The listing builds one solid part. Answer for the finished solid, in the listing's coordinates (mm). Face numbers are marked on the shaded views. A direction names the side the tool comes from. Give positions to 0.01 mm unless a question says otherwise; leave off trailing zeros. Loops run counter-clockwise (first coordinate to the right, second up) from the corner with the lowest first, then second, coordinate; pieces in that order, holes last. Notation, with made-up numbers: (86, -6.5) - (115, -6.5) arc R17 cw to (115, 2.5) - close; hole circle Ø2 at (39, -30.5). An arc over 180 degrees is marked (long way). One line per item, written item: value. Start each with the question number.
from build123d import *

# Parameters (mm, degrees)
SKETCH1_R           = 1.651
BOSS_EXTRUDE2_DEPTH = 6.35
SKETCH2_R           = 1.143
CUT_EXTRUDE1_DEPTH  = 7.35
SKETCH3_R           = 12.1285
CUT_EXTRUDE2_DEPTH  = 7.35
SKETCH4_W           = 28.562713242
SKETCH4_H           = 11.677503754
BOSS_EXTRUDE3_DEPTH = 6.35
SKETCH5_W           = 216.7214489
SKETCH5_H           = 130.569220634
CUT_EXTRUDE4_DEPTH  = 7.35
SKETCH11_R          = 3.937
CUT_EXTRUDE11_DEPTH = 7.35
SKETCH12_W          = 8.89
SKETCH12_H          = 8.89
CUT_EXTRUDE12_DEPTH = 7.35
SKETCH14_R          = 3.175
CUT_EXTRUDE14_DEPTH = 45.45
CUT_EXTRUDE15_DEPTH = 21.59
SKETCH16_R          = 12.192
CUT_EXTRUDE16_DEPTH = 21.59
SKETCH57_R          = 1.651
CUT_EXTRUDE57_DEPTH = 58.674


with BuildPart() as part:
    # Sketch1 → Boss-Extrude2 (new body)
    with BuildSketch(Plane.XY):
        with BuildLine():
            Line((-64.964441474, 37.338), (-54.550441474, 37.338))
            Line((-54.550441474, 37.338), (-54.550441474, -37.338))
            Line((-54.550441474, -37.338), (-64.964441474, -37.338))
            ThreePointArc((-64.964441474, -37.338), (0, -74.93), (64.964441474, -37.338))
            Line((64.964441474, -37.338), (54.550441474, -37.338))
            Line((54.550441474, -37.338), (54.550441474, 37.338))
            Line((54.550441474, 37.338), (64.964441474, 37.338))
            ThreePointArc((64.964441474, 37.338), (0, 74.93), (-64.964441474, 37.338))
        make_face()
        with Locations((-46.482, 11.049)):
            Circle(SKETCH1_R, mode=Mode.SUBTRACT)
        with Locations((-21.083270032, 10.795)):
            Circle(SKETCH1_R, mode=Mode.SUBTRACT)
        with Locations((-21.083270032, -10.795)):
            Circle(SKETCH1_R, mode=Mode.SUBTRACT)
        with Locations((-46.482, -11.049)):
            Circle(SKETCH1_R, mode=Mode.SUBTRACT)
        with Locations((46.482, -11.049)):
            Circle(SKETCH1_R, mode=Mode.SUBTRACT)
        with Locations((21.083270032, -10.795)):
            Circle(SKETCH1_R, mode=Mode.SUBTRACT)
        with Locations((21.083270032, 10.795)):
            Circle(SKETCH1_R, mode=Mode.SUBTRACT)
        with Locations((46.482, 11.049)):
            Circle(SKETCH1_R, mode=Mode.SUBTRACT)
    extrude(amount=BOSS_EXTRUDE2_DEPTH)

    # Sketch2 → Cut-Extrude1 (cut, through all)
    with BuildSketch(Plane.XY.offset(6.35)):
        with Locations((-6.731, 62.23)):
            Circle(SKETCH2_R)
        with Locations((6.731, 62.23)):
            Circle(SKETCH2_R)
    extrude(amount=-CUT_EXTRUDE1_DEPTH, mode=Mode.SUBTRACT)

    # Sketch3 → Cut-Extrude2 (cut, through all)
    with BuildSketch(Plane(origin=(0, 0, 0), x_dir=(-1, 0, 0), z_dir=(0, 0, -1))):
        with Locations((-15.777608989, -58.882838371)):
            Circle(SKETCH3_R)
        with Locations((15.777608989, -58.882838371)):
            Circle(SKETCH3_R)
        with Locations((-43.105229381, -43.105229381)):
            Circle(SKETCH3_R)
        with Locations((-43.105229381, 43.105229381)):
            Circle(SKETCH3_R)
        with Locations((43.105229381, 43.105229381)):
            Circle(SKETCH3_R)
        with Locations((43.105229381, -43.105229381)):
            Circle(SKETCH3_R)
    extrude(amount=-CUT_EXTRUDE2_DEPTH, mode=Mode.SUBTRACT)

    # Sketch4 → Boss-Extrude3 (add)
    with BuildSketch(Plane(origin=(0, 0, 0), x_dir=(-1, 0, 0), z_dir=(0, 0, -1))):
        with Locations((-1.488809975, 62.152540216)):
            Rectangle(SKETCH4_W, SKETCH4_H)
    extrude(amount=-BOSS_EXTRUDE3_DEPTH)

    # Sketch5 → Cut-Extrude4 (cut, through all)
    with BuildSketch(Plane(origin=(0, 0, 0), x_dir=(-1, 0, 0), z_dir=(0, 0, -1))):
        with Locations((23.316688373, 48.139610317)):
            Rectangle(SKETCH5_W, SKETCH5_H)
    extrude(amount=-CUT_EXTRUDE4_DEPTH, mode=Mode.SUBTRACT)

    # Sketch11 → Cut-Extrude11 (cut, through all)
    with BuildSketch(Plane(origin=(0, 0, 0), x_dir=(-1, 0, 0), z_dir=(0, 0, -1))):
        with Locations((0, -66.045)):
            Circle(SKETCH11_R)
    extrude(amount=-CUT_EXTRUDE11_DEPTH, mode=Mode.SUBTRACT)

    # Sketch12 → Cut-Extrude12 (cut, through all)
    with BuildSketch(Plane(origin=(0, 0, 0), x_dir=(-1, 0, 0), z_dir=(0, 0, -1))):
        with Locations((-33.605441474, -21.59)):
            Rectangle(SKETCH12_W, SKETCH12_H)
        with Locations((33.605441474, -21.59)):
            Rectangle(SKETCH12_W, SKETCH12_H)
    extrude(amount=-CUT_EXTRUDE12_DEPTH, mode=Mode.SUBTRACT)

    # Sketch14 → Cut-Extrude14 (cut, through all)
    with BuildSketch(Plane(origin=(30.092005081, 4.08352975, -38.1), x_dir=(-1, 0, 0), z_dir=(0, 0, -1))):
        with Locations((73.272005081, -29.48352975)):
            Circle(SKETCH14_R)
        with Locations((30.092005081, -29.48352975)):
            Circle(SKETCH14_R)
        with Locations((-13.087994919, -29.48352975)):
            Circle(SKETCH14_R)
    extrude(amount=-CUT_EXTRUDE14_DEPTH, mode=Mode.SUBTRACT)

    # Sketch15 → Cut-Extrude15 (cut)
    with BuildSketch(Plane(origin=(0, 0, 0), x_dir=(-1, 0, 0), z_dir=(0, 0, -1))):
        with BuildLine():
            Line((-12.7, -20.24), (-6.06, -20.24))
            Line((-6.06, -20.24), (12.7, -20.24))
            ThreePointArc((12.7, -20.24), (16.235533906, -11.704466094), (7.7, -15.24))
            Line((7.7, -15.24), (-1.06, -15.24))
            ThreePointArc((-1.06, -15.24), (-4.010609847, -10.6792983), (-9.38, -11.501337137))
            ThreePointArc((-9.38, -11.501337137), (-17.374040774, -13.464234575), (-12.7, -20.24))
        make_face()
    extrude(amount=-CUT_EXTRUDE15_DEPTH, mode=Mode.SUBTRACT)

    # Sketch16 → Cut-Extrude16 (cut)
    with BuildSketch(Plane(origin=(0, 0, 0), x_dir=(-1, 0, 0), z_dir=(0, 0, -1))):
        with Locations((15.777608989, -33.482838371)):
            Circle(SKETCH16_R)
        with Locations((-15.777608989, -33.482838371)):
            Circle(SKETCH16_R)
    extrude(amount=-CUT_EXTRUDE16_DEPTH, mode=Mode.SUBTRACT)

    # Sketch57 → Cut-Extrude57 (cut)
    with BuildSketch(Plane(origin=(0, 0, 0), x_dir=(-1, 0, 0), z_dir=(0, 0, -1))):
        with Locations((-25.937608989, -45.645229381)):
            Circle(SKETCH57_R)
        with Locations((25.937608989, -45.645229381)):
            Circle(SKETCH57_R)
    extrude(amount=-CUT_EXTRUDE57_DEPTH, mode=Mode.SUBTRACT)


solid = part.part
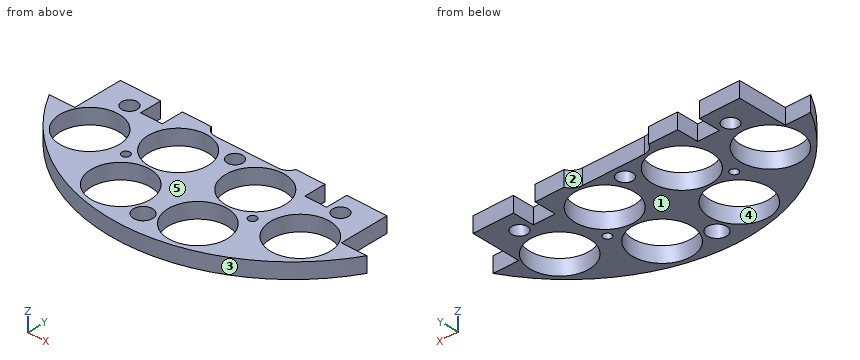
1. Determine the mould class of the marked faces 3, 4 and 5 for opening direction Y: released by +Y, released by -Y, zero draft, split by the parting line, or undercut.
2. A cutting plane is placed at B-B (y = -64.5). Determine the outline of the cut face in (x, z), plus the area to 3 significant figures.
3. For the marked faces 1 and 2, determine the directions among +Z, -Z, +X, -X, +Y, -Y from which every point of the face is accessible in a straight line to the end or side of a thin tool.
4. A cutting plane is placed at A-A (x = 0). Determine the outline of the cut face in (y, z) (3 decimals).
5. A cutting plane is placed at C-C (z = 1.75). Give the number of separate pieces and of enclosed holes in the cut face, plus the area to 3 significant figures.
6. Find the intervals of material crossed by L1, parallel to Y at x = -15.5, z = 2.75; L2, parallel to Y at x = 40.5, z = 0.75 (3 decimals); L3, parallel to X at y = -60, z = 1.25, in increasing order. Write a range as [from, to].
7. A cutting plane is placed at D-D (x = 19.5). Determine the outline of the cut face in (y, z) (3 decimals), plus the area to 3 significant figures.
8. Flat-ended cylindrical pins translate along their axes: pin 1 (2 mm diameter, centred on y = -33, z = 5.5, fed in from +X); pin 2 (3 mm diameter, centred on x = 35.5, z = 3, fed in from +Y) (3 decimals); pin 3 (3 mm diameter, centred on x = -57.5, z = 4.5, fed in from +Y). Find the tip coordinate at first contact, or state that the pin passes through.
Results below:
1. face 3: released by -Y
1. face 4: undercut
1. face 5: zero draft
2. outline: (-38.13, 0) - (-26.53, 0) - (-26.53, 6.35) - (-38.13, 6.35) - close; (-5.03, 0) - (-3.62, 0) - (-3.62, 6.35) - (-5.03, 6.35) - close; (3.62, 0) - (5.03, 0) - (5.03, 6.35) - (3.62, 6.35) - close; (26.53, 0) - (38.13, 0) - (38.13, 6.35) - (26.53, 6.35) - close
2. area: 165 mm^2
3. face 1: -Z, +X, -X, +Y, -Y
3. face 2: +Z, -Z, +Y
4. outline: (-74.93, 0) - (-69.982, 0) - (-69.982, 6.35) - (-74.93, 6.35) - close; (-62.108, 0) - (-28.575, 0) - (-28.575, 6.35) - (-62.108, 6.35) - close; (-22.225, 0) - (-20.24, 0) - (-20.24, 6.35) - (-22.225, 6.35) - close
5. separate pieces: 1
5. enclosed holes: 12
5. area: 2,470 mm^2
6. L1: y = [-73.31, -71.01], [-46.76, -45.67], [-21.29, -19.38]
6. L2: y = [-63.042, -54.951], [-31.26, -27.102], [-23.698, -17.145]
6. L3: x = [-44.88, -27.85], [-3.7, 3.7], [27.85, 44.88]
7. outline: (-72.348, 0) - (-70.426, 0) - (-70.426, 6.35) - (-72.348, 6.35) - close; (-47.34, 0) - (-45.093, 0) - (-45.093, 6.35) - (-47.34, 6.35) - close; (-21.873, 0) - (-17.145, 0) - (-17.145, 6.35) - (-21.873, 6.35) - close
7. area: 56.5 mm^2
8. pin 1: stops at x = 54.55
8. pin 2: stops at y = -26.035
8. pin 3: stops at y = -37.34
